Check sheet for the modelled part. Datum: model origin and axes. Units: mm. A direction names the side the tool comes from. Coordinates: 2 decimals unless noted, no trailing zeros. Order: outer loops, then holes, each group sorted by start corner. A loop starts at its lowest first (then second) coordinate and runs counter-clockwise, first axis right, second up.
from build123d import *

# Parameters (mm, degrees)
SKETCH2_R               = 4.3
BOSS_EXTRUDE2_DEPTH     = 57.08
CUT_EXTRUDE2_DEPTH      = 21.08
SKETCH6_R               = 0.6
CUT_EXTRUDE3_DEPTH      = 5.3
CUT_EXTRUDE3_DEPTH_BACK = 5.3
SKETCH7_R               = 0.6
CUT_EXTRUDE4_DEPTH      = 10
SKETCH8_R               = 0.6
CUT_EXTRUDE5_DEPTH      = 5.3000001
CUT_EXTRUDE5_DEPTH_BACK = 5.3000001
SKETCH9_R               = 0.6
CUT_EXTRUDE6_DEPTH      = 7.4500001


with BuildPart() as part:
    # Sketch2 → Boss-Extrude2 (new body)
    with BuildSketch(Plane(origin=(0, 0, 0), x_dir=(1, 0, 0), z_dir=(0, 1, 0))):
        Circle(SKETCH2_R)
    extrude(amount=BOSS_EXTRUDE2_DEPTH)

    # Sketch4 → Cut-Extrude2 (cut)
    with BuildSketch(Plane(origin=(0, 57.08, 0), x_dir=(1, 0, 0), z_dir=(0, 1, 0))):
        with BuildLine():
            Line((0, 2.15), (-3.723909236, 2.15))
            ThreePointArc((-3.723909236, 2.15), (0, 4.3), (3.723909236, 2.15))
            Line((3.723909236, 2.15), (0, 2.15))
        make_face()
        with BuildLine():
            Line((0, -2.15), (-3.723909236, -2.15))
            ThreePointArc((-3.723909236, -2.15), (0, -4.3), (3.723909236, -2.15))
            Line((3.723909236, -2.15), (0, -2.15))
        make_face()
    extrude(amount=-CUT_EXTRUDE2_DEPTH, mode=Mode.SUBTRACT)

    # Sketch6 → Cut-Extrude3 (cut, two sides)
    with BuildSketch(Plane.XY) as cut_extrude3_sk:
        with Locations((0, 1.5)):
            Circle(SKETCH6_R)
    extrude(amount=CUT_EXTRUDE3_DEPTH, mode=Mode.SUBTRACT)
    extrude(cut_extrude3_sk.sketch, amount=-CUT_EXTRUDE3_DEPTH_BACK, mode=Mode.SUBTRACT)

    # Sketch7 → Cut-Extrude4 (cut)
    with BuildSketch(Plane.XY.offset(2.15)):
        with Locations((0, 38)):
            Circle(SKETCH7_R)
    extrude(amount=-CUT_EXTRUDE4_DEPTH, mode=Mode.SUBTRACT)

    # Sketch8 → Cut-Extrude5 (cut, two sides)
    with BuildSketch(Plane.XY) as cut_extrude5_sk:
        with Locations((0, 20)):
            Circle(SKETCH8_R)
    extrude(amount=CUT_EXTRUDE5_DEPTH, mode=Mode.SUBTRACT)
    extrude(cut_extrude5_sk.sketch, amount=-CUT_EXTRUDE5_DEPTH_BACK, mode=Mode.SUBTRACT)

    # Sketch9 → Cut-Extrude6 (cut, through all)
    with BuildSketch(Plane.XY.offset(2.15)):
        with Locations((0, 52.5)):
            Circle(SKETCH9_R)
    extrude(amount=-CUT_EXTRUDE6_DEPTH, mode=Mode.SUBTRACT)


solid = part.part
(1) Thickness scan on probe 1 along Y at (x, z) = (0, 1); probe 2 along Y at (x, z) = (0, -2.5); probe 3 along Y at (x, z) = (-0.25, -2.25). Record the ranges inside material, lowest first.
Filled in:
probe 1: y = 0 to 0.9, 2.1 to 19.4, 20.6 to 37.4, 38.6 to 51.9, 53.1 to 57.08
probe 2: y = 0 to 0.9, 2.1 to 19.4, 20.6 to 36
probe 3: y = 0 to 0.95, 2.05 to 19.45, 20.55 to 36
(2) Cross-section at C-C (z = -1.5). Enter the section's corners in (x, y), and give its area (3 significant figures).
Filled in:
outline: (-4.03, 0) - (4.03, 0) - (4.03, 57.08) - (-4.03, 57.08) - close; hole circle Ø1.2 at (0, 1.5); hole circle Ø1.2 at (0, 20); hole circle Ø1.2 at (0, 38); hole circle Ø1.2 at (0, 52.5)
area: 456 mm2
(3) Go/stop test with flat-tipped pins: P1, Ø3.5, axis at x = 0, y = 50.5, coming from the -Z side; P2, Ø1, axis at y = 18.5, z = -2.5, coming from the +X side; P3, Ø1, axis at y = 48, z = -2.5, coming from the -X side. Record where each tip stops, or that it passes through.
Filled in:
P1: stops at z = -2.15
P2: stops at x = 3.81
P3: stops at x = -3.81
(4) Cross-section at B-B (y = 38). Enter the section's corners in (x, z), and give its area (3 significant figures).
Filled in:
outline: (-3.72, -2.15) - (-0.6, -2.15) - (-0.6, 2.15) - (-3.72, 2.15) arc R4.3 ccw to start; (0.6, -2.15) - (3.72, -2.15) arc R4.3 ccw to (3.72, 2.15) - (0.6, 2.15) - close
area: 30.2 mm2
(5) Cross-section at D-D (y = 47). Enter the section's corners in (x, z).
Filled in:
outline: (-3.72, -2.15) - (3.72, -2.15) arc R4.3 ccw to (3.72, 2.15) - (-3.72, 2.15) arc R4.3 ccw to start
(6) Tool access check on faces 1 (the flat face through (0, 36, 3)), 2 (the cylindrical face through (-0.13, 51.914, 0.03)), 3 (the flat face through (0, 36, -3)). Record the directions out of +Z, -Z, +X, -X, +Y, -Y that give a thin tool (end or side, any length) a straight path to the whole face; none if there is none.
Filled in:
face 1: +Z, +X, -X, +Y
face 2: +Z, -Z
face 3: -Z, +X, -X, +Y
(7) Release check for a two-part mould opening along Y. For faces 4 (the cylindrical face through (-0.078, 38.595, 0.03)), 5 (the flat face through (0, 57.08, 0)), 6 (the flat face through (0, 47, -2.15)) record: +Y half, -Y half, draft (parallel to the pull), parting line (faces both ways), or undercut.
Filled in:
face 4: undercut
face 5: +Y half
face 6: draft
(8) Cross-section at A-A (x = 0). Enter the section's corners in (y, z).
Filled in:
outline: (0, -4.3) - (0.9, -4.3) - (0.9, 4.3) - (0, 4.3) - close; (2.1, -4.3) - (19.4, -4.3) - (19.4, 4.3) - (2.1, 4.3) - close; (20.6, -4.3) - (36, -4.3) - (36, -2.15) - (37.4, -2.15) - (37.4, 2.15) - (36, 2.15) - (36, 4.3) - (20.6, 4.3) - close; (38.6, -2.15) - (51.9, -2.15) - (51.9, 2.15) - (38.6, 2.15) - close; (53.1, -2.15) - (57.08, -2.15) - (57.08, 2.15) - (53.1, 2.15) - close
